from build123d import *

# Parameters (mm, degrees)
SKETCH1_W           = 21.7
SKETCH1_H           = 17.7
BOSS_EXTRUDE1_DEPTH = 4.125
SKETCH3_OUTSIDE_W   = 29.538
SKETCH3_OUTSIDE_H   = 25.538
CUT_EXTRUDE1_DEPTH  = 8.25


with BuildPart() as part:
    # Sketch1 → Boss-Extrude1 (new, symmetric)
    with BuildSketch(Plane.XY):
        with Locations((0, 8.85)):
            Rectangle(SKETCH1_W, SKETCH1_H)
    extrude(amount=BOSS_EXTRUDE1_DEPTH, both=True)

    # Sketch3 outside → Cut-Extrude1 (cut)
    with BuildSketch(Plane.XY.offset(4.125)):
        with Locations((0, 8.85)):
            Rectangle(SKETCH3_OUTSIDE_W, SKETCH3_OUTSIDE_H)
        with BuildLine():
            Line((-4.75, 17.7), (4.75, 17.7))
            ThreePointArc((4.75, 17.7), (19.75, 2.7), (4.75, -12.3))
            Line((4.75, -12.3), (-4.75, -12.3))
            ThreePointArc((-4.75, -12.3), (-19.75, 2.7), (-4.75, 17.7))
        make_face(mode=Mode.SUBTRACT)
    extrude(amount=-CUT_EXTRUDE1_DEPTH, mode=Mode.SUBTRACT)

    # Sketch5 → CBORE for M2.5 SHCS1 (revolve, cut)
    with BuildSketch(Plane(origin=(0, 17.7, 0.575), x_dir=(0, 0, 1), z_dir=(1, 0, 0))):
        Polygon((0, 0), (0, 17.7), (1.45, 17.7), (1.45, 12.5), (2.75, 12.5), (2.75, 0.025), (2.775, 0), align=None)
    revolve(axis=Axis((0, 24.05, 0.575), (0, -1, 0)), mode=Mode.SUBTRACT)


solid = part.part
The listing builds one solid part. Answer for the finished solid, in the listing's coordinates (mm). A direction names the side the tool comes from. Coordinates: 2 decimals unless noted, no trailing zeros. Write each loop counter-clockwise with the first axis right and the second up, starting at its lowest first coordinate (ties: lowest second). Pieces come first, ordered by that corner, then holes. Notation, with made-up numbers: M -5.5,0.25 L 47.5,0.25 A14 ccw 47.5,7.25 Z; hole C 57,17 d10. An arc over 180 degrees is marked long. Use one line per item in the form item = value.
Item 1: Find section A-A, the plane x = 0. Give the vertices of the cut face in (y, z) (3 decimals).
Model answer:
outline = M 0,-4.125 L 17.7,-4.125 L 17.7,-2.2 L 17.675,-2.175 L 5.2,-2.175 L 5.2,-0.875 L 0,-0.875 Z; M 0,2.025 L 5.2,2.025 L 5.2,3.325 L 17.675,3.325 L 17.7,3.35 L 17.7,4.125 L 0,4.125 Z
Item 2: Find section D-D, the plane x = 7.75. Give the vertices of the cut face in (y, z) (3 decimals), plus the area to 3 significant figures.
Model answer:
outline = M 0,-4.125 L 17.397,-4.125 L 17.397,4.125 L 0,4.125 Z
area = 144 mm2
Item 3: For faces 4 (the face through (1, 5.2, -1)), 5 (the face through (10.85, 8, 0)), determine the directions among +Z, -Z, +X, -X, +Y, -Y from which every point of the face is accessible in a straight line to the end or side of a thin tool.
Model answer:
face_4 = +Y
face_5 = +Z, -Z, +X, +Y, -Y
Item 4: Find section B-B, the plane y = 4.25. Give the vertices of the cut face in (x, z) (3 decimals).
Model answer:
outline = M -10.85,-4.125 L 10.85,-4.125 L 10.85,4.125 L -10.85,4.125 Z; hole C 0,0.575 d2.9
Item 5: The mould has two halves that part along Z. Classify faces 1 (the face through (-0.436, 2.636, 1.958)), 2 (the face through (-10.85, 8, 0)), 3 (the face through (0, 9, 4.125)): released by +Z, released by -Z, zero draft, split by the parting line, or undercut.
Model answer:
face_1 = undercut
face_2 = zero draft
face_3 = released by +Z
Item 6: Given P1, Ø4, axis at x = 0, z = 0.575, coming from the +Y side, flat-ended and moving along its own axis, determine where the tip first touches the part or whether it passes through.
Model answer:
P1 = 5.2
Item 7: Find the intervals of material crossed by probe 1 along X at (y, z) = (5.25, 0.5); probe 2 along Z at (x, y) = (0, 2.3) (3 decimals); probe 3 along Z at (x, y) = (0, 9.25) (3 decimals), in increasing order.
Model answer:
probe_1 = -10.85 to -2.75, 2.75 to 10.85
probe_2 = -4.125 to -0.875, 2.025 to 4.125
probe_3 = -4.125 to -2.175, 3.325 to 4.125
Item 8: Find section C-C, the plane y = 11. Give the vertices of the cut face in (x, z) (3 decimals).
Model answer:
outline = M -10.85,-4.125 L 10.85,-4.125 L 10.85,4.125 L -10.85,4.125 Z; hole C 0,0.575 d5.5
